Read the model definition and answer for the solid it produces. Units are mm, in the model's axes. Face numbers are marked on the shaded views. A direction names the side the tool comes from. Give positions to 0.01 mm unless a question says otherwise; leave off trailing zeros. Loops run counter-clockwise (first coordinate to the right, second up) from the corner with the lowest first, then second, coordinate; pieces in that order, holes last. Notation, with made-up numbers: (27, 56) - (59, 56) arc R14 ccw to (59, 62) - close; hole circle Ø8 at (68, -26). An arc over 180 degrees is marked (long way). Write each question's results on one line, items separated by ' | '. Start each with the question number.
Q1. The part is cut by section A-A, the plane y = 9.5. Write down the section's boundary in (x, z).
Q2. Find the intervals of material crossed by line 1 (Y direction, x = 2.5, z = -9.5); line 2 (Z direction, x = 3, y = 10); line 3 (Y direction, x = 8.5, z = -12), in increasing order. Write a range as from..to.
Q3. For the marked faces 5, 6 and 7, determine the directions among +Z, -Z, +X, -X, +Y, -Y from which every point of the face is accessible in a straight line to the end or side of a thin tool.
Q4. The part is cut by section D-D, the plane y = 25. Write down the section's boundary in (x, z), plus the area to 3 significant figures.
Q5. Determine the mould class of the marked faces 1, 2, 3 and 4 for opening direction Z: +Z half, -Z half, draft (parallel to the pull), parting line (faces both ways), or undercut.
Q6. Given pin 1 (3 mm diameter, centred on x = 5.5, y = 17, fed in from +Z); pin 2 (8 mm diameter, centred on x = 8, y = 25, fed in from -Z); pin 3 (2 mm diameter, centred on x = -5.5, y = 16, fed in from -Z), each flat-ended and moving along its own axis, determine where each tip first touches the part or whether it passes through.
Q7. The part is cut by section C-C, the plane y = 29. Write down the section's boundary in (x, z), plus the area to 3 significant figures.
Q8. The part is cut by section B-B, the plane z = 0. Write down the section's boundary in (x, y), plus the area to 3 significant figures.
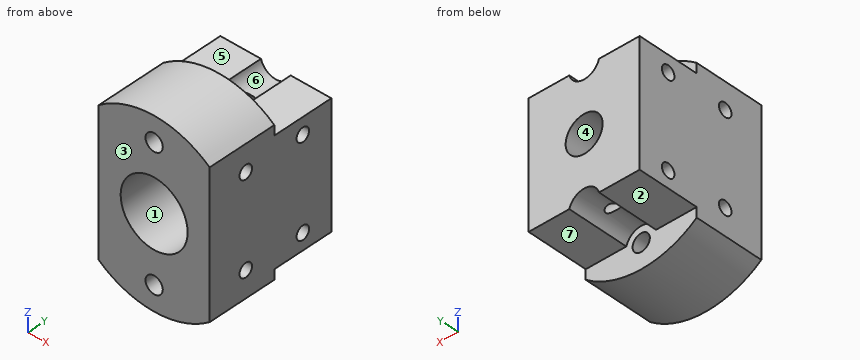
```python
from build123d import *

# Parameters (mm, degrees)
SKETCH_1_R          = 2.1
SKETCH_1_R_2        = 8.15
EXTRUDE_1_DEPTH     = 17
SKETCH_2_W          = 27
SKETCH_2_H          = 30
EXTRUDE_2_DEPTH     = 15
SKETCH_3_R          = 3.75
CUT_EXTRUDE_2_DEPTH = 15
SKETCH_4_R          = 1.65
CUT_EXTRUDE_3_DEPTH = 48.296934362
SKETCH_5_R          = 4.5
CUT_EXTRUDE_4_DEPTH = 42.112650154


with BuildPart() as part:
    # 草图1 → 凸台-拉伸1 (new body)
    with BuildSketch(Plane(origin=(0, 0, 0), x_dir=(1, 0, 0), z_dir=(0, 1, 0))):
        with BuildLine():
            Line((-13.5, -17.370952766), (-13.5, 17.370952766))
            ThreePointArc((-13.5, 17.370952766), (0, 22), (13.5, 17.370952766))
            Line((13.5, 17.370952766), (13.5, -17.370952766))
            ThreePointArc((13.5, -17.370952766), (0, -22), (-13.5, -17.370952766))
        make_face()
        with Locations(Location((0, 16, 0), (0, 0, 270))):
            Circle(SKETCH_1_R, mode=Mode.SUBTRACT)
        with Locations(Location((0, -16, 0), (0, 0, 270))):
            Circle(SKETCH_1_R, mode=Mode.SUBTRACT)
        with Locations(Location((0, 0, 0), (0, 0, 270))):
            Circle(SKETCH_1_R_2, mode=Mode.SUBTRACT)
    extrude(amount=EXTRUDE_1_DEPTH)

    # 草图2 → 凸台-拉伸2 (add)
    with BuildSketch(Plane(origin=(0, 17, 0), x_dir=(1, 0, 0), z_dir=(0, 1, 0))):
        Rectangle(SKETCH_2_W, SKETCH_2_H)
    extrude(amount=EXTRUDE_2_DEPTH)

    # 草图3 → 切除-拉伸2 (cut)
    with BuildSketch(Plane(origin=(0, 32, 0), x_dir=(1, 0, 0), z_dir=(0, 1, 0))):
        with Locations((0, 16)):
            Circle(SKETCH_3_R)
        with Locations((0, -16)):
            Circle(SKETCH_3_R)
    extrude(amount=-CUT_EXTRUDE_2_DEPTH, mode=Mode.SUBTRACT)

    # 草图4 → 切除-拉伸3 (cut, through all)
    with BuildSketch(Plane.ZY.offset(13.5)):
        with Locations((11, 24.5)):
            Circle(SKETCH_4_R)
        with Locations(Location((-11, 24.5, 0), (0, 0, 180))):
            Circle(SKETCH_4_R)
        with Locations((11, 9.5)):
            Circle(SKETCH_4_R)
        with Locations(Location((-11, 9.5, 0), (0, 0, 180))):
            Circle(SKETCH_4_R)
    extrude(amount=-CUT_EXTRUDE_3_DEPTH, mode=Mode.SUBTRACT)

    # 草图5 → 切除-拉伸4 (cut, through all)
    with BuildSketch(Plane(origin=(0, 32, 0), x_dir=(1, 0, 0), z_dir=(0, 1, 0))):
        with Locations(Location((0, 0, 0), (0, 0, 270))):
            Circle(SKETCH_5_R)
    extrude(amount=-CUT_EXTRUDE_4_DEPTH, mode=Mode.SUBTRACT)


solid = part.part
```
Check sheet entries:
1) outline: (-13.5, -17.37) arc R22 ccw to (13.5, -17.37) - (13.5, -12.65) - (-13.5, -12.65) - close; (-13.5, -9.35) - (13.5, -9.35) - (13.5, 9.35) - (-13.5, 9.35) - close; (-13.5, 12.65) - (13.5, 12.65) - (13.5, 17.37) arc R22 ccw to (-13.5, 17.37) - close; hole circle Ø16.3 at (0, 0); hole circle Ø4.2 at (0, -16); hole circle Ø4.2 at (0, 16)
2) line 1: y = 0..8.81, 10.19..23.81, 25.19..32 | line 2: z = -21.79..-12.57, -9.43..-7.58, 7.58..9.43, 12.57..21.79 | line 3: y = 0..8.19, 10.81..23.19, 25.81..32
3) face 5: +Z, +X, -X, +Y | face 6: +Z, +Y | face 7: -Z, +X, -X, +Y
4) outline: (-13.5, -15) - (-3.61, -15) arc R3.75 cw to (-1.52, -12.57) - (-13.5, -12.57) - close; (-13.5, -9.43) - (13.5, -9.43) - (13.5, 9.43) - (-13.5, 9.43) - close; (-13.5, 12.57) - (-1.52, 12.57) arc R3.75 cw to (-3.61, 15) - (-13.5, 15) - close; (1.52, -12.57) arc R3.75 cw to (3.61, -15) - (13.5, -15) - (13.5, -12.57) - close; (1.52, 12.57) - (13.5, 12.57) - (13.5, 15) - (3.61, 15) arc R3.75 cw to start; hole circle Ø9 at (0, 0) | area: 549 mm^2
5) face 1: undercut | face 2: -Z half | face 3: draft | face 4: undercut
6) pin 1: stops at z = 21.63 | pin 2: stops at z = -15 | pin 3: stops at z = -21.53
7) outline: (-13.5, -15) - (-3.61, -15) arc R3.75 cw to (3.61, -15) - (13.5, -15) - (13.5, 15) - (3.61, 15) arc R3.75 cw to (-3.61, 15) - (-13.5, 15) - close; hole circle Ø9 at (0, 0) | area: 717 mm^2
8) outline: (-13.5, 0) - (-8.15, 0) - (-8.15, 17) - (-4.5, 17) - (-4.5, 32) - (-13.5, 32) - close; (4.5, 17) - (8.15, 17) - (8.15, 0) - (13.5, 0) - (13.5, 32) - (4.5, 32) - close | area: 452 mm^2
